Input: dimensioned drawing with shaded views. Units: mm. Origin: part minimum x, y, z. A direction names the side the tool comes from. Coordinates: 2 decimals unless noted, no trailing zeros. Write each loop counter-clockwise with the first axis right and the second up, starting at its lowest first coordinate (ties: lowest second). Pieces come first, ordered by that corner, then holes. Notation, with made-up numbers: M 6,78 L 24,78 A31 cw 24,106 Z; hole C 24,-3 d10. An arc over 180 degrees is marked long. Use one line per item in the form item = value.
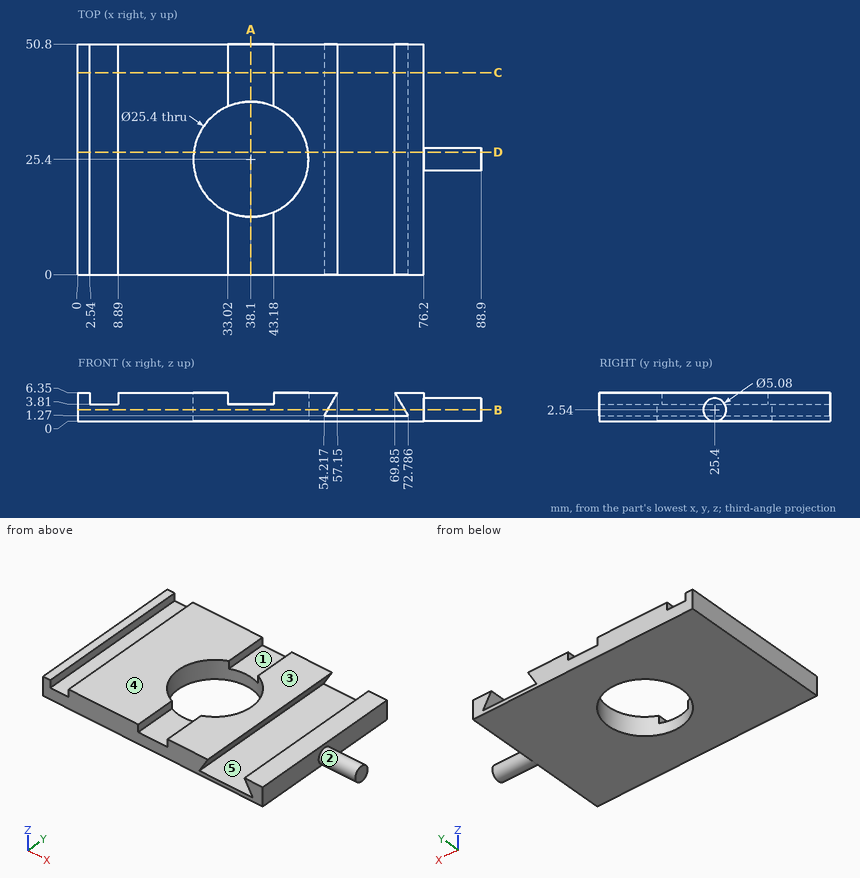
(1) Set-up query: the marked faces 1, 2 and 3. Return all of +Z, -Z, +X, -X, +Y, -Y with unobstructed straight access to the full face (end or side cutting, diameter ignored); none if empty.
Computed:
face_1 = +Z, +Y, -Y
face_2 = +X
face_3 = +Z, +X, -X, +Y, -Y
(2) Section query A-A on x = 38.1. Return the cut outline in (y, z).
Computed:
outline = M 0,0 L 12.7,0 L 12.7,3.81 L 0,3.81 Z; M 38.1,0 L 50.8,0 L 50.8,3.81 L 38.1,3.81 Z
(3) Section query C-C on y = 44.5. Return the cut outline in (x, z), plus the area to 4 significant figures.
Computed:
outline = M 0,0 L 76.2,0 L 76.2,6.35 L 69.85,6.35 L 72.79,1.27 L 54.22,1.27 L 57.15,6.35 L 43.18,6.35 L 43.18,3.81 L 33.02,3.81 L 33.02,6.35 L 8.89,6.35 L 8.89,3.81 L 2.54,3.81 L 2.54,6.35 L 0,6.35 Z
area = 362.5 mm^2
(4) Pull-direction query (X, two-part tool) for the marked faces 4 and 5; classes: pulls with the +X half, pulls with the -X half, needs draft (parallel to the pull), parting line crosses it, or undercut.
Computed:
face_4 = needs draft
face_5 = undercut
(5) Line query: probe 1 along X at (y, z) = (38, 5); probe 2 along X at (y, z) = (33.5, 2.5) (1 decimal); probe 3 along Y at (x, z) = (38.1, 3). Output: solid intervals per line, ascending.
Computed:
probe_1 = 0 to 2.54, 8.89 to 33.02, 43.18 to 56.37, 70.63 to 76.2
probe_2 = 0 to 28.3, 47.9 to 54.9, 72.1 to 76.2
probe_3 = 0 to 12.7, 38.1 to 50.8
(6) Section query D-D on y = 27. Return the cut outline in (x, z).
Computed:
outline = M 0,0 L 25.5,0 L 25.5,6.35 L 8.89,6.35 L 8.89,3.81 L 2.54,3.81 L 2.54,6.35 L 0,6.35 Z; M 50.7,0 L 76.2,0 L 76.2,0.57 L 88.9,0.57 L 88.9,4.51 L 76.2,4.51 L 76.2,6.35 L 69.85,6.35 L 72.79,1.27 L 54.22,1.27 L 57.15,6.35 L 50.7,6.35 Z
(7) Section query B-B on z = 2.54. Return the cut outline in (x, y), plus the area to 3 significant figures.
Computed:
outline = M 0,0 L 54.95,0 L 54.95,50.8 L 0,50.8 Z; M 72.05,0 L 76.2,0 L 76.2,22.86 L 88.9,22.86 L 88.9,27.94 L 76.2,27.94 L 76.2,50.8 L 72.05,50.8 Z; hole C 38.1,25.4 d25.4
area = 2,560 mm^2
(8) First-contact query: pin 1 Ø1.5 at (y, z) = (41, 2) entering from +X; pin 2 Ø1.9 at (x, y) = (5.5, 13) entering from +Z. Flat tips, straight axial feed; report the tip coordinate or a pass-through.
Computed:
pin_1 = 76.2
pin_2 = 3.81
